Geometry: final body of the model. Coordinates: model frame, mm. Face numbers are marked on the shaded views. A direction names the side the tool comes from. Coordinates: 2 decimals unless noted, no trailing zeros. Write each loop counter-clockwise with the first axis right and the second up, starting at its lowest first coordinate (ties: lowest second). Pieces come first, ordered by that corner, then holes. Notation, with made-up numbers: (18.5, 44.5) - (25.5, 44.5) arc R18 ccw to (25.5, 71.5) - close; hole circle Ø9 at (71, -32.5). An arc over 180 degrees is marked (long way). Answer as a JSON object with one key per item and string values. Group by question number.
Item 1: Mould query, pull axis Z, two halves, no side actions, for the marked faces 3, 4, 5 and 6. Classes: pulls with the +Z half, pulls with the -Z half, needs draft (parallel to the pull), parting line crosses it, or undercut.
Item 2: Line query: line 1 along Y through (x, z) = (-12, -23.5); line 2 along X through (y, z) = (20.5, 8); line 3 along X through (y, z) = (22, 4). Output: solid intervals per line, ascending. Write a range as from..to.
Item 3: Section A-A on z = 0. Return loops of the section in (x, y) (3 decimals).
Item 4: Section C-C on x = -10.16. Return loops of the section in (y, z) (1 decimal), and give its area (3 significant figures).
Item 5: Set-up query: the marked faces 1 and 2. Return all of +Z, -Z, +X, -X, +Y, -Y with unobstructed straight access to the full face (end or side cutting, diameter ignored); none if empty.
Item 6: Section D-D on z = -9.5. Return loops of the section in (x, y), and give its area (3 significant figures).
Item 7: First-contact query: pin 1 Ø12 at (x, y) = (19, 29.5) entering from +Z; pin 2 Ø1.5 at (y, z) = (16, -20.5) entering from +X; pin 3 Ø3 at (x, y) = (-24, 34) entering from -Z; pin 4 Ø4 at (x, z) = (0, -10.16) entering from -Y. Flat tips, straight axial feed; report the tip coordinate or a pass-through.
Item 8: Section B-B on x = 0. Return loops of the section in (y, z) (3 decimals).
```python
from build123d import *

# Parameters (mm, degrees)
SKETCH1_R                            = 31.75
BOSS_EXTRUDE1_DEPTH                  = 63.5
CUT_EXTRUDE2_START                   = -25.4
SKETCH2_R                            = 31.75
SKETCH2_R_2                          = 24.765
CUT_EXTRUDE2_DEPTH                   = 25.4
SKETCH3_R                            = 15.875
CUT_EXTRUDE3_DEPTH                   = 50.8
F_1_4_0_25_DIAMETER_HOLE1_AT_2_COUNT = 2
F_1_4_0_25_DIAMETER_HOLE1_AT_2_PITCH = 10.16
CIRPATTERN1_COUNT                    = 4


with BuildPart() as part:
    # Sketch1 → Boss-Extrude1 (new body)
    with BuildSketch(Plane(origin=(0, 0, 0), x_dir=(1, 0, 0), z_dir=(0, 1, 0))):
        with Locations(Location((0, 0, 0), (0, 0, 270))):
            Circle(SKETCH1_R)
    extrude(amount=BOSS_EXTRUDE1_DEPTH)

    # Sketch2 → Cut-Extrude2 (cut)
    with BuildSketch(Plane(origin=(0, 63.5, 0), x_dir=(1, 0, 0), z_dir=(0, 1, 0)).offset(CUT_EXTRUDE2_START)):
        with Locations(Location((0, 0, 0), (0, 0, 270))):
            Circle(SKETCH2_R)
        with Locations(Location((0, 0, 0), (0, 0, 270))):
            Circle(SKETCH2_R_2, mode=Mode.SUBTRACT)
    extrude(amount=CUT_EXTRUDE2_DEPTH, mode=Mode.SUBTRACT)

    # Sketch3 → Cut-Extrude3 (cut)
    with BuildSketch(Plane(origin=(0, 63.5, 0), x_dir=(1, 0, 0), z_dir=(0, 1, 0))):
        with Locations(Location((0, 0, 0), (0, 0, 270))):
            Circle(SKETCH3_R)
    extrude(amount=-CUT_EXTRUDE3_DEPTH, mode=Mode.SUBTRACT)

    # Sketch9 → 1/4 (0.25) Diameter Hole1 (revolve, cut)
    with BuildSketch(Plane(origin=(0, 0, -10.16), x_dir=(0, 0, -1), z_dir=(1, 0, 0))):
        Polygon((0, 0), (0, 14.607732465), (3.175, 12.7), (3.175, 0), align=None)
    f_1_4_0_25_diameter_hole1 = revolve(axis=Axis((0, -6.35, -10.16), (0, 1, 0)), mode=Mode.SUBTRACT)

    # 1/4 (0.25) Diameter Hole1 at 2: 1/4 (0.25) Diameter Hole1 ×2
    with Locations(*[(0, 0, i * F_1_4_0_25_DIAMETER_HOLE1_AT_2_PITCH) for i in range(1, F_1_4_0_25_DIAMETER_HOLE1_AT_2_COUNT)]):
        add(f_1_4_0_25_diameter_hole1, mode=Mode.SUBTRACT)

    # CirPattern1: 1/4 (0.25) Diameter Hole1 ×4 about axis
    cirpattern1_axis = Axis((0, 0, 0), (0, 1, 0))
    for i in range(1, CIRPATTERN1_COUNT):
        add(f_1_4_0_25_diameter_hole1.rotate(cirpattern1_axis, i * 360 / CIRPATTERN1_COUNT), mode=Mode.SUBTRACT)

    # CirPattern1 copy 1 sketch → CirPattern1 copy 1 (revolve, cut)
    with BuildSketch(Plane(origin=(0, 0, 0), x_dir=(-1, 0, 0), z_dir=(0, 0, -1))):
        Polygon((0, 0), (0, 14.607732465), (3.175, 12.7), (3.175, 0), align=None)
    revolve(axis=Axis((0, -6.35, 0), (0, 1, 0)), mode=Mode.SUBTRACT)

    # CirPattern1 copy 2 sketch → CirPattern1 copy 2 (revolve, cut)
    with BuildSketch(Plane.ZY):
        Polygon((0, 0), (0, 14.607732465), (3.175, 12.7), (3.175, 0), align=None)
    revolve(axis=Axis((0, -6.35, 0), (0, 1, 0)), mode=Mode.SUBTRACT)

    # CirPattern1 copy 3 sketch → CirPattern1 copy 3 (revolve, cut)
    with BuildSketch(Plane.XY):
        Polygon((0, 0), (0, 14.607732465), (3.175, 12.7), (3.175, 0), align=None)
    revolve(axis=Axis((0, -6.35, 0), (0, 1, 0)), mode=Mode.SUBTRACT)


solid = part.part
```
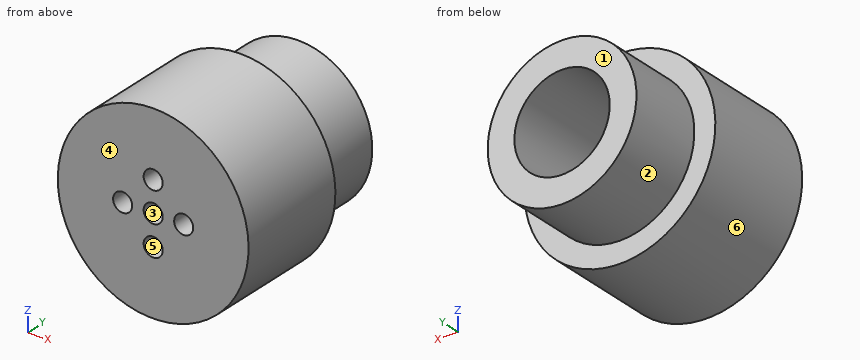
Checks:
{
 "1": {"face 3": "undercut", "face 4": "needs draft", "face 5": "undercut", "face 6": "parting line crosses it"},
 "2": {"line 1": "0..38.1", "line 2": "-30.73..-13.71, 13.71..30.73", "line 3": "-31.5..-15.36, 15.36..31.5"},
 "3": {"outline": "(-31.75, 0) - (-13.335, 0) - (-13.335, 12.7) - (-15.875, 12.7) - (-15.875, 63.5) - (-24.765, 63.5) - (-24.765, 38.1) - (-31.75, 38.1) - close; (-6.985, 0) - (-3.175, 0) - (-3.175, 12.7) - (-6.985, 12.7) - close; (3.175, 0) - (6.985, 0) - (6.985, 12.7) - (3.175, 12.7) - close; (13.335, 0) - (31.75, 0) - (31.75, 38.1) - (24.765, 38.1) - (24.765, 63.5) - (15.875, 63.5) - (15.875, 12.7) - (13.335, 12.7) - close"},
 "4": {"outline": "(0, -30.1) - (38.1, -30.1) - (38.1, -22.6) - (63.5, -22.6) - (63.5, -12.2) - (12.7, -12.2) - (12.7, -3.2) - (0, -3.2) - close; (0, 3.2) - (12.7, 3.2) - (12.7, 12.2) - (63.5, 12.2) - (63.5, 22.6) - (38.1, 22.6) - (38.1, 30.1) - (0, 30.1) - close", "area": "2,120 mm^2"},
 "5": {"face 1": "+Z, -Z, +X, -X, +Y", "face 2": "+Y"},
 "6": {"outline": "(-30.3, 0) - (-3.11, 0) - (-3.11, 12.7) - (-12.72, 12.7) - (-12.72, 63.5) - (-22.87, 63.5) - (-22.87, 38.1) - (-30.3, 38.1) - close; (3.11, 0) - (30.3, 0) - (30.3, 38.1) - (22.87, 38.1) - (22.87, 63.5) - (12.72, 63.5) - (12.72, 12.7) - (3.11, 12.7) - close", "area": "2,100 mm^2"},
 "7": {"pin 1": "z = 28.97", "pin 2": "x = 24.86", "pin 3": "z = -22.4", "pin 4": "through"},
 "8": {"outline": "(0, -31.75) - (38.1, -31.75) - (38.1, -24.765) - (63.5, -24.765) - (63.5, -15.875) - (12.7, -15.875) - (12.7, -13.335) - (0, -13.335) - close; (0, -6.985) - (12.7, -6.985) - (12.7, -3.175) - (0, -3.175) - close; (0, 3.175) - (12.7, 3.175) - (12.7, 6.985) - (0, 6.985) - close; (0, 13.335) - (12.7, 13.335) - (12.7, 15.875) - (63.5, 15.875) - (63.5, 24.765) - (38.1, 24.765) - (38.1, 31.75) - (0, 31.75) - close"}
}
